Part print with two shaded views. Sizes in mm from the minimum x, y, z corner. Round coordinates to 2 decimals unless told otherwise and drop trailing zeros. Order: outer loops, then holes, each group sorted by start corner. A loop starts at its lowest first (then second) coordinate and runs counter-clockwise, first axis right, second up. Notation, with made-up numbers: (57, -34) - (68, -34) arc R33 ccw to (68, 2) - close; hole circle Ø7 at (75.5, 31). An arc over 180 degrees is marked (long way). Write item = value, one per line.
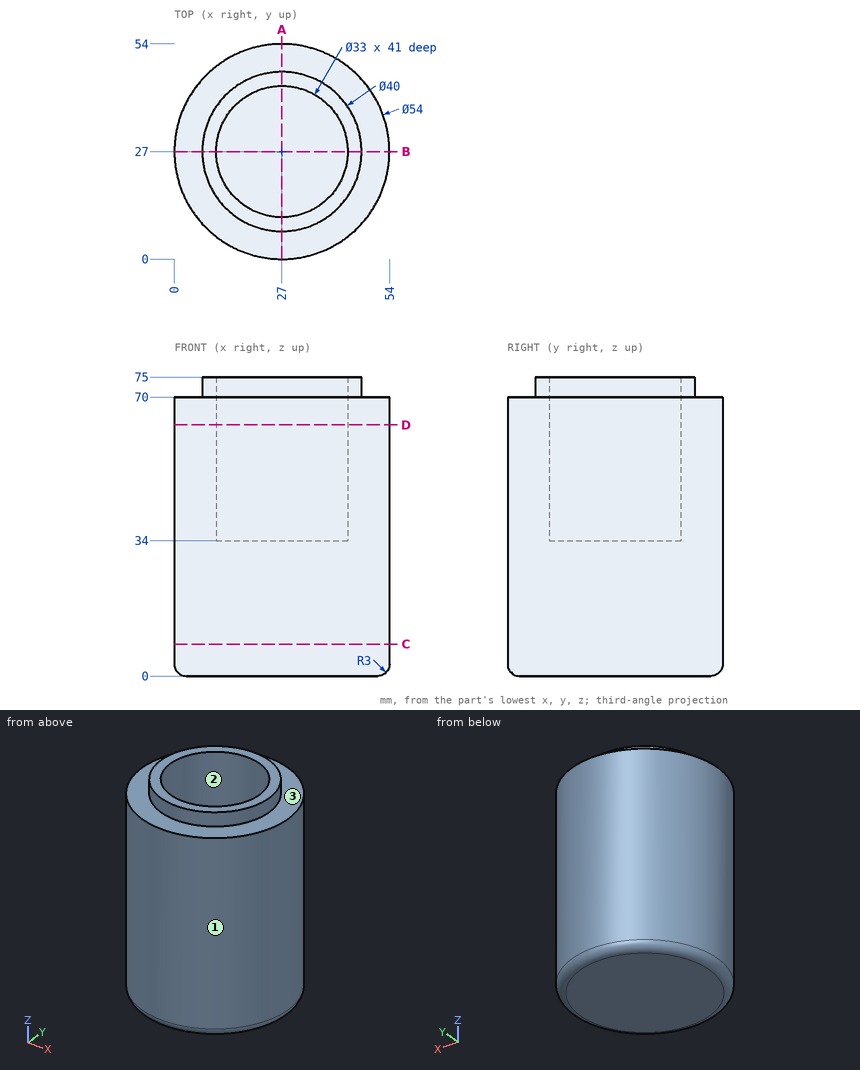
1) Mould opens along Y. For the marked faces 1, 2 and 3 say: +Y half, -Y half, draft (parallel to the pull), parting line (faces both ways), or undercut.
Conclusion:
face_1 = parting line
face_2 = undercut
face_3 = draft
2) Cut at D-D (z = 63). Write the cut outline in (x, y).
Conclusion:
outline = circle Ø54 at (27, 27); hole circle Ø33 at (27, 27)
3) Wall check: line 1 along Y through (x, z) = (27, 49); line 2 along Z through (x, y) = (38.5, 38); line 3 along X through (y, z) = (22.5, 40.5). Give the ranges that are in metal, low to high.
Conclusion:
line_1 = 0 to 10.5, 43.5 to 54
line_2 = 0 to 34
line_3 = 0.38 to 11.13, 42.87 to 53.62
4) Cut at A-A (x = 27). Write the cut outline in (y, z), and give its area (3 significant figures).
Conclusion:
outline = (0, 3) arc R3 ccw to (3, 0) - (51, 0) arc R3 ccw to (54, 3) - (54, 70) - (47, 70) - (47, 75) - (43.5, 75) - (43.5, 34) - (10.5, 34) - (10.5, 75) - (7, 75) - (7, 70) - (0, 70) - close
area = 2,620 mm^2
5) Cut at C-C (z = 8). Write the cut outline in (x, y).
Conclusion:
outline = circle Ø54 at (27, 27)
6) Flat gauge pins, fed straight in: pin 1 Ø2 at (y, z) = (34, 61) entering from +X; pin 2 Ø3 at (y, z) = (32.5, 42.5) entering from +X; pin 3 Ø4 at (x, z) = (47.5, 55) entering from +Y. Where does each tip first touch, or does it go through?
Conclusion:
pin_1 = 53.32
pin_2 = 53.7
pin_3 = 46.67
